Can you work these out from the model? Positions are in its coordinate system, mm. A direction names the side the tool comes from. Give positions to 0.01 mm unless a question says otherwise; leave off trailing zeros. Write each loop counter-clockwise with the first axis right and the second up, starting at its lowest first coordinate (ties: lowest second). Pieces come first, ordered by that corner, then holes. Notation, with made-up numbers: (-39, 84.5) -> (-24, 84.5) arc R25 ccw to (-24, 98.5) -> close; hole circle Ø11 at (0, 42). An arc over 180 degrees is marked (long way). Answer as CSV lines item,"result". Start each with the question number.
1. I'm going to push flat-ended pins straight in: P1, Ø1, axis at x = 1.5, z = -1.5, coming from the -Y side; P2, Ø1.5, axis at x = 1.5, z = -2, coming from the +Y side. Where does each tip first touch, or does it pass through?
2. If we section it at A-A on y = -3.75: Write out the boundary of the cut face in (x, z).
3. If we mould it in two halves opening along X, with no side actions, what happens to faces 1 (the face through (-1.5, -4.79, -0.07)), 2 (the face through (0, -10, 0)), 3 (the face through (0.469, 0.507, -0.895))? For each: pulls with the +X half, pulls with the -X half, needs draft (parallel to the pull), parting line crosses it, or undercut.
4. On a 3-axis mill with a long thin cutter (end or side, diameter ignored), from which of +Z, -Z, +X, -X, +Y, -Y can I reach the whole of each face in a straight line? I mean faces 4 (the face through (-1.2, 0, 1.2)), 5 (the face through (-1.01, 0.51, 0.04)), 6 (the face through (-2.44, 0.15, 1.27)). Say none if no direction works.
5. I need wall thicknesses on line 1 (Y direction, x = -0.3, z = -0.3); line 2 (X direction, y = 0.25, z = 0.4); line 3 (X direction, y = -7.75, z = 0). Which ranges of each line are inside material? Lowest first, please. Write a range as [from, to].
```python
from build123d import *

# Parameters (mm, degrees)
SKETCH1_R           = 2.75
BOSS_EXTRUDE1_DEPTH = 0.3
SKETCH2_R           = 1.25
CUT_EXTRUDE1_DEPTH  = 1


# Read off the part's stored shape, not the designer's step: M3x0.5 Machine Threads Stud1
with BuildPart() as part:
    # Sketch1 → Boss-Extrude1 (new body)
    with BuildSketch(Plane(origin=(0, 0, 0), x_dir=(1, 0, 0), z_dir=(0, 1, 0))):
        with Locations(Location((0, 0, 0), (0, 0, 270))):
            Circle(SKETCH1_R)
    extrude(amount=BOSS_EXTRUDE1_DEPTH)

    # Sketch2 → section 0 of loft1
    with BuildSketch(Plane(origin=(0, 1, 0), x_dir=(1, 0, 0), z_dir=(0, 1, 0)), mode=Mode.PRIVATE) as loft1_s0:
        Circle(SKETCH2_R)
    # loft up to a face of the part (loft1)
    loft([loft1_s0.sketch, Face(Wire([part.edges().sort_by_distance((2.004663725, 0.3, -1.882504541))[0]]))])

    # Sketch2<4> → Cut-Extrude1 (cut)
    with BuildSketch(Plane(origin=(0, 1, 0), x_dir=(1, 0, 0), z_dir=(0, 1, 0))):
        Polygon((-0.98095369, -0.632504307), (0.057287953, -1.165782969), (1.038241642, -0.533278662), (0.98095369, 0.632504307), (-0.057287953, 1.165782969), (-1.038241642, 0.533278662), align=None)
    extrude(amount=-CUT_EXTRUDE1_DEPTH, mode=Mode.SUBTRACT)

    # M3x0.5 Machine Threads Stud1 outline → M3x0.5 Machine Threads Stud1 (revolve)
    with BuildSketch(Plane.XY):
        Polygon((0, 0), (0, -10), (1.2195, -10), (1.5, -9.7195), (1.5, 0), align=None)
    revolve(axis=Axis((0, 0, 0), (0, 1, 0)))


solid = part.part
```
Computed values:
1,P1,"stops at y = 0"
1,P2,"stops at y = 0.77"
2,outline,"circle Ø3 at (0, 0)"
3,face 1,"parting line crosses it"
3,face 2,"needs draft"
3,face 3,"undercut"
4,face 4,"-Y"
4,face 5,"+Y"
4,face 6,"+Y, -Y"
5,line 1,"y = [-10, 0]"
5,line 2,"x = [-2.72, -0.99], [1.03, 2.72]"
5,line 3,"x = [-1.5, 1.5]"
